Check sheet for the modelled part. Datum: model origin and axes. Units: mm. Give positions to 0.01 mm unless a question says otherwise; leave off trailing zeros. Order: outer loops, then holes, each group sorted by start corner. A loop starts at its lowest first (then second) coordinate and runs counter-clockwise, first axis right, second up.
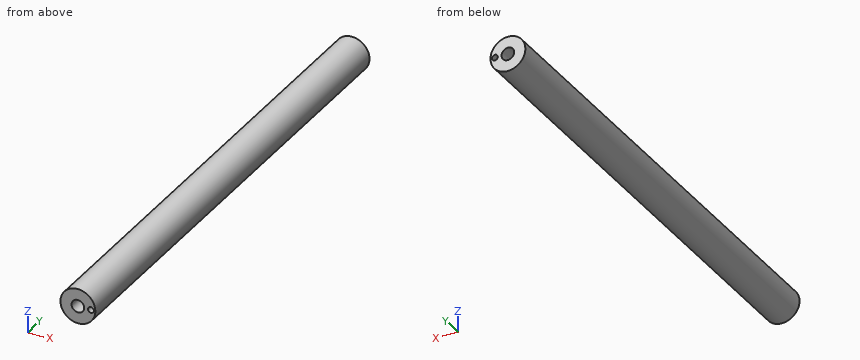
```python
from build123d import *

# Parameters (mm, degrees)
SKETCH1_R                                    = 4.7625
BOSS_EXTRUDE1_DEPTH                          = 133.35
F_8_32_TAPPED_HOLE1_D                        = 3.4544
F_8_32_TAPPED_HOLE1_DEPTH                    = 10.668
F_8_32_TAPPED_HOLE1_TIP                      = 1.037806461
F_8_32_TAPPED_HOLE1_ON_FACE_2_D              = 3.4544
F_8_32_TAPPED_HOLE1_ON_FACE_2_DEPTH          = 10.668
F_8_32_TAPPED_HOLE1_ON_FACE_2_TIP            = 1.037806461
F_1_16_0_0625_DIAMETER_HOLE1_D               = 1.5875
F_1_16_0_0625_DIAMETER_HOLE1_DEPTH           = 4.7625
F_1_16_0_0625_DIAMETER_HOLE1_TIP             = 0.476933116
F_1_16_0_0625_DIAMETER_HOLE1_ON_FACE_2_D     = 1.5875
F_1_16_0_0625_DIAMETER_HOLE1_ON_FACE_2_DEPTH = 4.7625
F_1_16_0_0625_DIAMETER_HOLE1_ON_FACE_2_TIP   = 0.476933116


with BuildPart() as part:
    # Sketch1 → Boss-Extrude1 (new body)
    with BuildSketch(Plane(origin=(0, 0, 0), x_dir=(1, 0, 0), z_dir=(0, 1, 0))):
        with Locations(Location((0, 0, 0), (0, 0, 270))):
            Circle(SKETCH1_R)
    extrude(amount=BOSS_EXTRUDE1_DEPTH)

    # #8-32 Tapped Hole1
    with Locations(Plane.ZX.offset(133.35)):
        with Locations((0, 0)):
            Hole(F_8_32_TAPPED_HOLE1_D / 2, depth=F_8_32_TAPPED_HOLE1_DEPTH)
            with Locations((0, 0, -(F_8_32_TAPPED_HOLE1_DEPTH + F_8_32_TAPPED_HOLE1_TIP / 2))):  # 118° drill point
                Cone(0, F_8_32_TAPPED_HOLE1_D / 2, F_8_32_TAPPED_HOLE1_TIP, mode=Mode.SUBTRACT)

    # #8-32 Tapped Hole1 on face 2
    with Locations(Plane(origin=(0, 0, 0), x_dir=(0, 0, -1), z_dir=(0, -1, 0))):
        with Locations((0, 0)):
            Hole(F_8_32_TAPPED_HOLE1_ON_FACE_2_D / 2, depth=F_8_32_TAPPED_HOLE1_ON_FACE_2_DEPTH)
            with Locations((0, 0, -(F_8_32_TAPPED_HOLE1_ON_FACE_2_DEPTH + F_8_32_TAPPED_HOLE1_ON_FACE_2_TIP / 2))):  # 118° drill point
                Cone(0, F_8_32_TAPPED_HOLE1_ON_FACE_2_D / 2, F_8_32_TAPPED_HOLE1_ON_FACE_2_TIP, mode=Mode.SUBTRACT)

    # 1/16 (0.0625) Diameter Hole1
    with Locations(Plane(origin=(3.556, 0, 0), x_dir=(0, 0, -1), z_dir=(0, -1, 0))):
        with Locations((0, 0)):
            Hole(F_1_16_0_0625_DIAMETER_HOLE1_D / 2, depth=F_1_16_0_0625_DIAMETER_HOLE1_DEPTH)
            with Locations((0, 0, -(F_1_16_0_0625_DIAMETER_HOLE1_DEPTH + F_1_16_0_0625_DIAMETER_HOLE1_TIP / 2))):  # 118° drill point
                Cone(0, F_1_16_0_0625_DIAMETER_HOLE1_D / 2, F_1_16_0_0625_DIAMETER_HOLE1_TIP, mode=Mode.SUBTRACT)

    # 1/16 (0.0625) Diameter Hole1 on face 2
    with Locations(Plane(origin=(3.556, 133.35, 0), x_dir=(0, 0, 1), z_dir=(0, 1, 0))):
        with Locations((0, 0)):
            Hole(F_1_16_0_0625_DIAMETER_HOLE1_ON_FACE_2_D / 2, depth=F_1_16_0_0625_DIAMETER_HOLE1_ON_FACE_2_DEPTH)
            with Locations((0, 0, -(F_1_16_0_0625_DIAMETER_HOLE1_ON_FACE_2_DEPTH + F_1_16_0_0625_DIAMETER_HOLE1_ON_FACE_2_TIP / 2))):  # 118° drill point
                Cone(0, F_1_16_0_0625_DIAMETER_HOLE1_ON_FACE_2_D / 2, F_1_16_0_0625_DIAMETER_HOLE1_ON_FACE_2_TIP, mode=Mode.SUBTRACT)


solid = part.part
```
(1) Sectioned sample at A-A (y = 124). Enter the section's corners in (x, z) (1 decimal).
(2) Thickness scan on L1, parallel to X at y = 132, z = 0; L2, parallel to X at y = 7.5, z = 0; L3, parallel to X at y = 51, z = 0.25. Record the ranges inside material, lowest first.
(3) Go/stop test with flat-tipped pins: P1, Ø4, axis at x = 0.5, z = 0.5, coming from the +Y side; P2, Ø3, axis at x = 0, z = 0, coming from the -Y side; P3, Ø5, axis at x = 4, y = 69.5, coming from the +Z side. Record where each tip stops, or that it passes through.
(4) Sectioned sample at B-B (y = 108.5). Enter the section's corners in (x, z) (1 decimal).
Values follow:
1. outline: circle Ø9.5 at (0, 0); hole circle Ø3.5 at (0, 0)
2. L1: x = -4.76 to -1.73, 1.73 to 2.76, 4.35 to 4.76
2. L2: x = -4.76 to -1.73, 1.73 to 4.76
2. L3: x = -4.76 to 4.76
3. P1: stops at y = 133.35
3. P2: stops at y = 10.8
3. P3: stops at z = 4.52
4. outline: circle Ø9.5 at (0, 0)
